from build123d import *

# Parameters (mm, degrees)
F6_R           = 2.286
F8_DEPTH       = 9.35
F9_SIZE        = 0.3
F10_R          = 4.7503425206
F11_DEPTH      = 0.75
F11_DEPTH_BACK = 0.75


# Not quite as in the source:
# - a fillet or chamfer that OpenCascade refuses, or shapes differently, is made with other operations: its cross-section is extruded or revolved along the edge and cut away or added
# - the program builds the solid bodies; features that only make, move or delete a surface that nothing else refers to are left out


with BuildPart() as f8:
    # F6 (on Right) → F8 (new body)
    with BuildSketch(Plane.YZ):
        Circle(F6_R)
    extrude(amount=-F8_DEPTH)

    # F9
    f9_edges = [f8.edges().sort_by_distance(p)[0] for p in [
        (-9.35, -2.286, 0),
    ]]
    chamfer(f9_edges, length=F9_SIZE)

    # F10 (on Right) → F11 (join, two sides)
    with BuildSketch(Plane.YZ) as f11_sk:
        Circle(F10_R)
    extrude(amount=F11_DEPTH)
    extrude(f11_sk.sketch, amount=-F11_DEPTH_BACK)

    # F12: fillet of radius 2.2 on 1 edges, made by hand

    # F12_s1 → F12_t2 (revolve, cut)
    with BuildSketch(Plane.XY):
        with BuildLine():
            ThreePointArc((-0.75, 4.7503425206), (0.3360571099, 3.949200417), (0.75, 2.6646771591))
            Line((0.75, 2.6646771591), (0.75, 4.7503425206))
            Line((0.75, 4.7503425206), (-0.75, 4.7503425206))
        make_face()
    revolve(axis=Axis((0.75, 0, 0), (1, 0, 0)), mode=Mode.SUBTRACT)


solid = f8.part
Design review of the part built by this model. Coordinates are the model's own, in mm. A direction names the side the tool comes from. Round coordinates to 2 decimals unless told otherwise and drop trailing zeros. Loops run counter-clockwise (first coordinate to the right, second up) from the corner with the lowest first, then second, coordinate; pieces in that order, holes last. Notation, with made-up numbers: M 23,17.25 L 82,17.25 A20 ccw 82,40.25 Z; hole C 77,20 d10. An arc over 180 degrees is marked long. Answer as a JSON object with one key per item and string values.
Item 1: Machinability: for faces 1 (the flat face through (-9.35, 0, 0)), 2 (the cylindrical face through (-4.84, -0.5, -2.23)), which of the approach directions +Z, -Z, +X, -X, +Y, -Y give a long, thin tool a straight path to every point of the face, cutting with its end or side? Answer none if there is none.
Answer sheet:
{"face 1": "+Z, -Z, -X, +Y, -Y", "face 2": "-X"}
Item 2: We need section A-A on y = 0. Give the boundary of the cut face in (x, z), and give its area (3 significant figures).
Answer sheet:
{"outline": "M -9.35,-1.99 L -9.05,-2.29 L -0.75,-2.29 L -0.75,-4.75 A2.2 ccw 0.75,-2.66 L 0.75,2.66 A2.2 ccw -0.75,4.75 L -0.75,2.29 L -9.05,2.29 L -9.35,1.99 Z", "area": "51.8 mm^2"}
Item 3: Wall thickness on L1, parallel to X at y = -1.75, z = 2; L2, parallel to Z at x = -7, y = -1; L3, parallel to X at y = -1, z = -3.5: over which ranges is each line inside the solid? List them lowest first. Write a range as from..to.
Answer sheet:
{"L1": "x = -0.75..0.75", "L2": "z = -2.06..2.06", "L3": "x = -0.75..0.52"}
Item 4: Clearance check with flat-ended pins moving along their axes: P1, Ø3, axis at x = -0.5, z = -3.5, coming from the +Y side; P2, Ø2, axis at x = -4, z = 3.5, coming from the +Y side; P3, Ø5, axis at x = -4, y = 2, coming from the -Z side; P4, Ø3, axis at y = 1.5, z = -3.5, coming from the +X side. State where each tip first meets the part, or that it passes through.
Answer sheet:
{"P1": "stops at y = 4.3", "P2": "passes through", "P3": "stops at z = -2.29", "P4": "stops at x = 0.75"}
Item 5: We need section C-C on x = -2.5. Give the boundary of the cut face in (y, z).
Answer sheet:
{"outline": "C 0,0 d4.57"}
